For this review, take the finished solid that the model builds, in its own axes (mm). A direction names the side the tool comes from. Give positions to 0.01 mm unless a question says otherwise; leave off trailing zeros. Write each loop counter-clockwise with the first axis right and the second up, starting at its lowest first coordinate (ties: lowest second). Pieces come first, ordered by that corner, then holes.
1) Machinability: for faces 3 (the face through (76, 11.5, 55)), 4 (the face through (82.013, 3, 61)), which of the approach directions +Z, -Z, +X, -X, +Y, -Y give a long, thin tool a straight path to every point of the face, cutting with its end or side? Answer none if there is none.
2) We need section C-C on z = 49. Give the boundary of the cut face in (x, y), and give its area (3 significant figures).
3) We need section D-D on y = 9.25. Give the boundary of the cut face in (x, z).
4) Wall thickness on line 1 along X through (y, z) = (5.75, 58); line 2 along Z through (x, y) = (63, 8.25); line 3 along X through (y, z) = (8.5, 40): over which ranges is each line inside the solid? List them lowest first.
5) We need section A-A on y = 3.5. Give the boundary of the cut face in (x, z).
6) Draft analysis for pull direction Z (two halves, no side actions). For faces 1 (the face through (78.025, 8.373, 53.802)), 2 (the face through (76, 0, 51)), state which applies: pulls with the +Z half, pulls with the -Z half, needs draft (parallel to the pull), parting line crosses it, or undercut.
7) For P1, Ø4, axis at y = 8, z = 42.5, coming from the -X side; P2, Ø1.5, axis at y = 7.5, z = 56.5, coming from the +X side; P3, Ø1, axis at y = 4, z = 61, coming from the +X side; P4, Ø5, axis at x = 88, z = 58, coming from the -Y side, all flat-tipped, find the tip position at first contact; note any pin that passes through.
8) We need section B-B on x = 88. Give the boundary of the cut face in (y, z).
Solid Edge part; units mm, degrees
sketch "Sketch1" plane through (0, 0, 0) normal (0, -1, 0) x (1, 0, 0)
  circle A0 centre (80.5127, 55.3877) radius 22.5
extrude "Protrusion1" add sketch "Sketch1" against normal blind 10
sketch "Sketch2" plane through (80.5127, 10, 55.3877) normal (0, 1, 0) x (0, 0, -1)
  circle A0 centre (0, 0) radius 2.95
extrude "ExtrudedCutout_5" cut sketch "Sketch2" against normal blind 4
sketch "Sketch3" plane through (80.5127, 6, 55.3877) normal (0, 1, 0) x (-1, 0, 0)
  circle A0 centre (0, 0) radius 1.05
extrude "Cutout1" cut sketch "Sketch3" against normal up to next
sketch "Sketch4" plane through (80.5127, 5, 51.1598) normal (0, -1, 0) x (1, 0, 0)
  circle A0 centre (0, 4.2279) radius 3.55
extrude "ExtrudedCutout_7" cut sketch "Sketch4" against normal blind 0.5
chamfer "Chamfer_2" distance 1.9 distance2 0.5 1 edges at (80.5127, 6, 58.3377) measured on face at (78.605, 6, 53.362)
sketch "Sketch5" plane through (80.5127, 10, 55.3877) normal (0, 1, 0) x (0, 0, 1)
  circle A0 centre (0, 0) radius 22.5
  circle A1 centre (0, 0) radius 3
extrude "ExtrudedProtrusion_4" add sketch "Sketch5" along normal blind 1.5
sketch "Sketch6" plane through (80.5127, 0, 55.3877) normal (0, -1, 0) x (0, 0, 1)
  line L0 (-1.5, -5) -> (-1.5, -9.7)
  line L1 (-1.5, -9.7) -> (-2.5, -9.7)
  line L2 (-2.5, -9.7) -> (-2.5, -10.7)
  arc A0 (-2.5, -10.7) -> (2.4996, -10.6613) centre (0, -10.7) ccw
  line L3 (2.4996, -9.6613) -> (2.4996, -10.6613)
  line L4 (1.4996, -9.6613) -> (2.4996, -9.6613)
  line L5 (1.4996, -9.6613) -> (1.4996, -4.9613)
  arc A1 (1.4996, -4.9613) -> (5, -1.5) centre (1.4996, -1.4607) ccw
  line L6 (7, -1.5) -> (5, -1.5)
  arc A2 (7, 1.5) -> (7, -1.5) centre (7, 0) cw
  line L7 (5, 1.5) -> (7, 1.5)
  arc A3 (1.5, 5) -> (5, 1.5) centre (1.5, 1.5) cw
  line L8 (1.5, 7) -> (1.5, 5)
  arc A4 (-1.5, 7) -> (1.5, 7) centre (0, 7) cw
  line L9 (-1.5, 5) -> (-1.5, 7)
  arc A5 (-5, 1.5) -> (-1.5, 5) centre (-1.5, 1.5) cw
  line L10 (-5, 1.5) -> (-7, 1.5)
  arc A6 (-7, 1.5) -> (-7, -1.5) centre (-7, 0) ccw
  line L11 (-7, -1.5) -> (-5, -1.5)
  arc A7 (-5, -1.5) -> (-1.5, -5) centre (-1.5, -1.5) ccw
  dimension "D1" = 5
  dimension "D2" = 7
  dimension "D3" = 5
  dimension "D4" = 1.5
  dimension "D5" = 7
  dimension "D6" = 1.5
  dimension "D7" = 1.5
  dimension "D8" = 1.4996
  dimension "D9" = 2.4996
  dimension "D10" = 2.5
extrude "ExtrudedCutout_9" cut sketch "Sketch6" against normal blind 6.7
Results list:
1. face 3: +Z, -Z, +X, -X, +Y
1. face 4: -Y
2. outline: (58.94, 0) - (79.01, 0) - (79.01, 6.7) - (82.01, 6.7) - (82.01, 0) - (102.09, 0) - (102.09, 11.5) - (58.94, 11.5) - close
2. area: 476 mm2
3. outline: circle Ø45 at (80.51, 55.39); hole circle Ø5.9 at (80.51, 55.39)
4. line 1: x = 58.16 to 75.69, 85.29 to 102.86
4. line 2: z = 41.26 to 69.51
4. line 3: x = 64.1 to 96.93
5. outline: circle Ø45 at (80.51, 55.39); hole (73.51, 53.89) - (75.51, 53.89) arc R3.5 ccw to (79.01, 50.39) - (79.01, 48.39) arc R1.5 ccw to (82.01, 48.39) - (82.01, 50.39) arc R3.5 ccw to (85.51, 53.89) - (90.21, 53.89) - (90.21, 52.89) - (91.21, 52.89) arc R2.5 ccw (long way) to (91.17, 57.89) - (90.17, 57.89) - (90.17, 56.89) - (85.47, 56.89) arc R3.5 ccw to (82.01, 60.39) - (82.01, 62.39) arc R1.5 ccw to (79.01, 62.39) - (79.01, 60.39) arc R3.5 ccw to (75.51, 56.89) - (73.51, 56.89) arc R1.5 ccw to start
6. face 1: undercut
6. face 2: needs draft
7. P1: stops at x = 60.82
7. P2: stops at x = 103.01
7. P3: stops at x = 102.42
7. P4: stops at y = 0
8. outline: (0, 34.17) - (11.5, 34.17) - (11.5, 76.61) - (0, 76.61) - (0, 56.89) - (6.7, 56.89) - (6.7, 53.89) - (0, 53.89) - close
